from build123d import *

# Parameters (mm, degrees)
F0_R     = 19.05
F0_R_2   = 12.7
F1_DEPTH = 31.75
F2_DEPTH = 63.5
F3_R     = 2.54
F4_SIZE  = 3.81


with BuildPart() as f1:
    # F0 (on Top) → F1 (new body)
    with BuildSketch(Plane.XY):
        with BuildLine():
            ThreePointArc((7.9375, -37.2640053369), (29.6144284936, -23.970724332), (38.1, 0))
            ThreePointArc((38.1, 0), (29.6144284936, 23.970724332), (7.9375, 37.2640053369))
            ThreePointArc((7.9375, 37.2640053369), (-38.1, 0), (7.9375, -37.2640053369))
        make_face()
        Circle(F0_R, mode=Mode.SUBTRACT)
        with BuildLine():
            ThreePointArc((7.9375, 37.2640053369), (29.6144284936, 23.970724332), (38.1, 0))
            ThreePointArc((38.1, 0), (29.6144284936, -23.970724332), (7.9375, -37.2640053369))
            Line((7.9375, -37.2640053369), (80.8302083333, -21.7373364465))
            ThreePointArc((80.8302083333, -21.7373364465), (53.975, 0), (80.8302083333, 21.7373364465))
            Line((80.8302083333, 21.7373364465), (7.9375, 37.2640053369))
        make_face()
        with BuildLine():
            ThreePointArc((98.425, 0), (93.4750832879, 13.982922527), (80.8302083333, 21.7373364465))
            ThreePointArc((80.8302083333, 21.7373364465), (53.975, 0), (80.8302083333, -21.7373364465))
            ThreePointArc((80.8302083333, -21.7373364465), (93.4750832879, -13.982922527), (98.425, 0))
        make_face()
        with Locations((76.2, 0)):
            Circle(F0_R_2, mode=Mode.SUBTRACT)
    extrude(amount=F1_DEPTH)

    # F0 (on Top) → F2 (join)
    with BuildSketch(Plane.XY):
        with BuildLine():
            ThreePointArc((7.9375, -37.2640053369), (29.6144284936, -23.970724332), (38.1, 0))
            ThreePointArc((38.1, 0), (29.6144284936, 23.970724332), (7.9375, 37.2640053369))
            ThreePointArc((7.9375, 37.2640053369), (-38.1, 0), (7.9375, -37.2640053369))
        make_face()
        Circle(F0_R, mode=Mode.SUBTRACT)
    extrude(amount=F2_DEPTH)

    # F3
    f3_edges = [f1.edges().sort_by_distance(p)[0] for p in [
        (-7.9375, 37.264005, 63.5),
        (-19.05, 0, 63.5),
        (44.383854, -29.500671, 0),
    ]]
    fillet(f3_edges, radius=F3_R)

    # F4
    f4_edges = [f1.edges().sort_by_distance(p)[0] for p in [
        (-21.59, 0, 63.5),
        (63.5, 0, 31.75),
    ]]
    chamfer(f4_edges, length=F4_SIZE)


solid = f1.part
The model under review builds one solid part; all positions refer to its coordinate system, in mm. Give positions to 0.01 mm unless a question says otherwise; leave off trailing zeros. Order: outer loops, then holes, each group sorted by start corner. A loop starts at its lowest first (then second) coordinate and runs counter-clockwise, first axis right, second up. Notation, with made-up numbers: (50, 75) -> (84, 75) arc R19 ccw to (84, 81) -> close; hole circle Ø3 at (-18.5, -20). An arc over 180 degrees is marked (long way). Write item = value, one per line. Start each with the question number.
(1) For L1, parallel to Y at x = -0.5, z = 16; L2, parallel to X at y = 6.5, z = 28; L3, parallel to Y at x = 76.2, z = 21.5, list the stretches that pass through material, from the lowest coordinate up. Write a range as from..to.
(2) Take a section at B-B (z = 57.5). Write out the cut boundary in (x, y).
(3) Draft analysis for pull direction X (two halves, no side actions). For faces 1 (the flat face through (56, 0, 31.75)), 2 (the cylindrical face through (43.71, 28.86, 0.72)), 3 (the conical face through (83.13, 10.86, 28.12)), 4 (the cylindrical face through (-38.1, 0.3, 37.8)), state which applies: +X half, -X half, draft (parallel to the pull), parting line (faces both ways), or undercut.
(4) For pin 1 Ø1.5 at (x, y) = (39.5, -11.5) entering from +Z; pin 2 Ø4 at (y, z) = (21, 42) entering from +X; pin 3 Ø1.5 at (y, z) = (-2, 48) entering from -X, all flat-tipped, find the tip position at first contact; note any pin that passes through.
(5) Take a section at A-A (z = 14). State how many separate pieces and enclosed holes the cut face has, plus the area to 3 significant figures.
Returned:
q1.L1 = -38.1..-19.04, 19.04..38.1
q1.L2 = -37.54..-17.91, 17.91..65.22, 87.18..97.45
q1.L3 = -22.72..-12.7, 12.7..22.72
q2.outline = circle Ø76.2 at (0, 0); hole circle Ø38.1 at (0, 0)
q3.face_1 = draft
q3.face_2 = +X half
q3.face_3 = undercut
q3.face_4 = parting line
q4.pin_1 = 31.75
q4.pin_2 = 33.02
q4.pin_3 = -38.08
q5.separate_pieces = 1
q5.enclosed_holes = 2
q5.area = 6,110 mm²
